Read the model definition and answer for the solid it produces. Units are mm, in the model's axes. A direction names the side the tool comes from. Give positions to 0.01 mm unless a question says otherwise; leave off trailing zeros. Loops run counter-clockwise (first coordinate to the right, second up) from the corner with the lowest first, then second, coordinate; pieces in that order, holes last. Notation, with made-up numbers: (84.5, 77.25) -> (137.5, 77.25) arc R36 cw to (137.5, 114.25) -> close; hole circle Ø7 at (85, 12). An arc over 180 degrees is marked (long way). Write each question's results on one line, items separated by ' | '. Start each with the question number.
Item 1: Find the intervals of material crossed by line 1 (Z direction, x = 2.1, y = 57); line 2 (Y direction, x = 4.45, z = -6.5); line 3 (Z direction, x = 4.2, y = 53.5), in increasing order.
Item 2: Determine the mould class of faces 1 (the flat face through (4.753, 54.74, -11.274)), 2 (the flat face through (3, 4, 0)), 3 (the flat face through (3, 0, -7)) for opening direction Z: +Z half, -Z half, draft (parallel to the pull), parting line (faces both ways), or undercut.
Item 3: Section A-A on y = 42 is taken. Write down the section's boundary in (x, z).
Item 4: Section C-C on x = 2.85 is taken. State how many separate pieces and enclosed holes the cut face has, and give its area (3 significant figures).
Item 5: Which of the six approach directions +Z, -Z, +X, -X, +Y, -Y give full straight-line access (tool end or side, diameter ignored) to faces 4 (the flat face through (4.75, 32.01, -18.67)), 5 (the flat face through (3, 2, -38.75)), 6 (the flat face through (3, 23, -10)), 7 (the conical face through (4.642, 31.345, -9.544))?
Item 6: Section B-B on z = -23 is taken. Write down the section's boundary in (x, y), and give its area (3 significant figures).
Item 7: Each of these flat-tipped pins is pushed along its axis until it touches: P1, Ø3.5, axis at y = 60.63, z = -12.5, coming from the -X side; P2, Ø1.5, axis at x = 2.5, y = 24.5, coming from the +Z side; P3, Ø2.5, axis at x = 2, y = 2.5, coming from the +Z side. Where does it stop, or does it pass through?
```python
from build123d import *

# Parameters (mm, degrees)
SKETCH_1_R      = 1.575
SKETCH_1_R_2    = 1.5
EXTRUDE_1_DEPTH = 5
CHAMFER_1_SIZE  = 0.5
FILLET_1_R      = 1


with BuildPart() as part:
    # 草图1 → 凸台-拉伸1 (new body)
    with BuildSketch(Plane(origin=(5, 0, 0), x_dir=(0, 0, -1), z_dir=(1, 0, 0))):
        with BuildLine():
            Line((58.94037044, 21.690945588), (58.94037044, 28.938446994))
            ThreePointArc((58.94037044, 28.938446994), (58.369466934, 31.808572737), (56.743671299, 34.241747853))
            Line((56.743671299, 34.241747853), (45.79785286, 45.187566291))
            ThreePointArc((45.79785286, 45.187566291), (43.689786601, 49.341242238), (44.440461488, 53.938355946))
            ThreePointArc((44.440461488, 53.938355946), (43.535533906, 59.772215716), (37.701674136, 60.677143298))
            ThreePointArc((37.701674136, 60.677143298), (33.104560428, 59.926468411), (28.950884481, 62.03453467))
            Line((28.950884481, 62.03453467), (20.049497475, 70.935921677))
            ThreePointArc((20.049497475, 70.935921677), (18.281730522, 71.668154724), (16.513963569, 70.935921677))
            Line((16.513963569, 70.935921677), (-4.699239867, 49.722718241))
            ThreePointArc((-4.699239867, 49.722718241), (-5.431472914, 47.954951288), (-4.699239867, 46.187184335))
            Line((-4.699239867, 46.187184335), (7.803300859, 33.68464361))
            ThreePointArc((7.803300859, 33.68464361), (9.429096494, 31.251468493), (10, 28.381342751))
            Line((10, 28.381342751), (10, 17.5))
            ThreePointArc((10, 17.5), (7.803300859, 12.196699141), (2.5, 10))
            ThreePointArc((2.5, 10), (0.732233047, 9.267766953), (0, 7.5))
            Line((0, 7.5), (0, 0))
            Line((0, 0), (15, 0))
            Line((15, 0), (15, 5))
            Line((15, 5), (26.25, 5))
            Line((26.25, 5), (26.25, 0))
            Line((26.25, 0), (38.75, 0))
            Line((38.75, 0), (38.75, 5))
            Line((38.75, 5), (50, 5))
            Line((50, 5), (50, 0))
            Line((50, 0), (65, 0))
            Line((65, 0), (65, 12.5))
            ThreePointArc((65, 12.5), (64.587190878, 13.876093833), (63.48509261, 14.797736397))
            ThreePointArc((63.48509261, 14.797736397), (60.178797805, 17.562664088), (58.94037044, 21.690945588))
        make_face()
        with Locations(Location((40, 56.23668181, 0), (0, 0, 180))):
            Circle(SKETCH_1_R, mode=Mode.SUBTRACT)
        with Locations(Location((39.972231035, 19.370159659, 0), (0, 0, 180))):
            Circle(SKETCH_1_R_2, mode=Mode.SUBTRACT)
        with Locations(Location((12.501132586, 60.629840341, 0), (0, 0, 180))):
            Circle(SKETCH_1_R_2, mode=Mode.SUBTRACT)
        with Locations(Location((5.606841469, 53.735549225, 0), (0, 0, 180))):
            Circle(SKETCH_1_R_2, mode=Mode.SUBTRACT)
        with Locations(Location((46.866522151, 26.264450775, 0), (0, 0, 180))):
            Circle(SKETCH_1_R_2, mode=Mode.SUBTRACT)
        Polygon((19.165613998, 62.273863607), (48.510545417, 32.928932188), (33.307749622, 17.726136393), (3.962818203, 47.071067812), align=None, mode=Mode.SUBTRACT)
    extrude(amount=-EXTRUDE_1_DEPTH)

    # 倒角1
    chamfer_1_edges = [part.edges().sort_by_distance(p)[0] for p in [
        (0, 5, -44.375),
        (0, 2.5, -50),
        (0, 0, -57.5),
        (0, 6.25, -65),
        (0, 25.314696291, -58.94037044),
        (0, 31.808572737, -58.369466934),
        (0, 39.714657072, -51.27076208),
        (0, 49.341242238, -43.689786601),
        (5, 6.25, -65),
        (5, 0, -57.5),
        (5, 2.5, -50),
        (5, 5, -44.375),
        (5, 2.5, -38.75),
        (5, 0, -32.5),
        (0, 59.772215716, -43.535533906),
        (5, 2.5, -26.25),
        (5, 5, -20.625),
        (5, 2.5, -15),
        (5, 0, -7.5),
        (5, 3.75, 0),
        (5, 9.267766953, -0.732233047),
        (5, 12.196699141, -7.803300859),
        (5, 22.940671375, -10),
        (5, 31.251468493, -9.429096494),
        (5, 39.935913973, -1.552030496),
        (0, 59.926468411, -33.104560428),
        (5, 47.954951288, 5.431472914),
        (5, 60.329319959, -5.907361851),
        (5, 71.668154724, -18.281730522),
        (5, 66.485228174, -24.500190978),
        (5, 59.926468411, -33.104560428),
        (5, 59.772215716, -43.535533906),
        (5, 49.341242238, -43.689786601),
        (5, 39.714657072, -51.27076208),
        (5, 31.808572737, -58.369466934),
        (5, 25.314696291, -58.94037044),
        (0, 66.485228174, -24.500190978),
        (5, 17.562664088, -60.178797805),
        (5, 13.876093833, -64.587190878),
        (0, 71.668154724, -18.281730522),
        (0, 60.329319959, -5.907361851),
        (0, 47.954951288, 5.431472914),
        (0, 13.876093833, -64.587190878),
        (0, 39.935913973, -1.552030496),
        (0, 31.251468493, -9.429096494),
        (0, 22.940671375, -10),
        (0, 12.196699141, -7.803300859),
        (0, 56.23668181, -41.575),
        (5, 56.23668181, -41.575),
        (0, 9.267766953, -0.732233047),
        (0, 19.370159659, -41.472231035),
        (5, 19.370159659, -41.472231035),
        (0, 3.75, 0),
        (0, 0, -7.5),
        (0, 54.67246571, -11.5642161),
        (0, 47.601397898, -33.838079708),
        (0, 25.32753429, -40.90914752),
        (0, 32.398602102, -18.635283912),
        (5, 54.67246571, -11.5642161),
        (5, 32.398602102, -18.635283912),
        (5, 25.32753429, -40.90914752),
        (5, 47.601397898, -33.838079708),
        (0, 2.5, -15),
        (0, 5, -20.625),
        (0, 60.629840341, -14.001132586),
        (5, 60.629840341, -14.001132586),
        (0, 2.5, -26.25),
        (0, 17.562664088, -60.178797805),
        (0, 53.735549225, -7.106841469),
        (5, 53.735549225, -7.106841469),
        (0, 0, -32.5),
        (0, 26.264450775, -48.366522151),
        (5, 26.264450775, -48.366522151),
        (0, 2.5, -38.75),
    ]]
    chamfer(chamfer_1_edges, length=CHAMFER_1_SIZE)

    # 圆角1
    fillet_1_edges = [part.edges().sort_by_distance(p)[0] for p in [
        (2.5, 0, 0),
        (2.5, 0, -15),
        (2.5, 5, -15),
        (2.5, 5, -26.25),
        (2.5, 0, -26.25),
        (2.5, 0, -38.75),
        (2.5, 5, -38.75),
        (2.5, 5, -50),
        (2.5, 0, -50),
        (2.5, 0, -65),
    ]]
    fillet(fillet_1_edges, radius=FILLET_1_R)


solid = part.part
```
Findings:
1) line 1: -44.94 to -41.38, -38.62 to -24.44, -13.89 to -2.58 | line 2: 0 to 11.16, 34.99 to 44.53, 49.61 to 52.53, 54.94 to 60.92 | line 3: -44.23 to -27.94, -10.39 to -7.09, -4.13 to 0.92
2) face 1: undercut | face 2: +Z half | face 3: draft
3) outline: (0, -48.28) -> (0.5, -48.99) -> (4.5, -48.99) -> (5, -48.28) -> (5, -40.15) -> (4.5, -39.44) -> (0.5, -39.44) -> (0, -40.15) -> close; (0, -8.33) -> (0.5, -9.03) -> (4.5, -9.03) -> (5, -8.33) -> (5, -0.2) -> (4.5, 0.51) -> (0.5, 0.51) -> (0, -0.2) -> close
4) separate pieces: 1 | enclosed holes: 6 | area: 2,230 mm2
5) face 4: +X | face 5: +X, -X, -Y | face 6: +Z, +X, -X | face 7: +Z, +X
6) outline: (0, 5.5) -> (0.5, 5) -> (4.5, 5) -> (5, 5.5) -> (5, 27.33) -> (4.5, 28.03) -> (0.5, 28.03) -> (0, 27.33) -> close; (0, 59.15) -> (0.5, 58.44) -> (4.5, 58.44) -> (5, 59.15) -> (5, 67.28) -> (4.5, 67.99) -> (0.5, 67.99) -> (0, 67.28) -> close | area: 162 mm2
7) P1: x = 0.25 | P2: z = -10 | P3: z = 0
